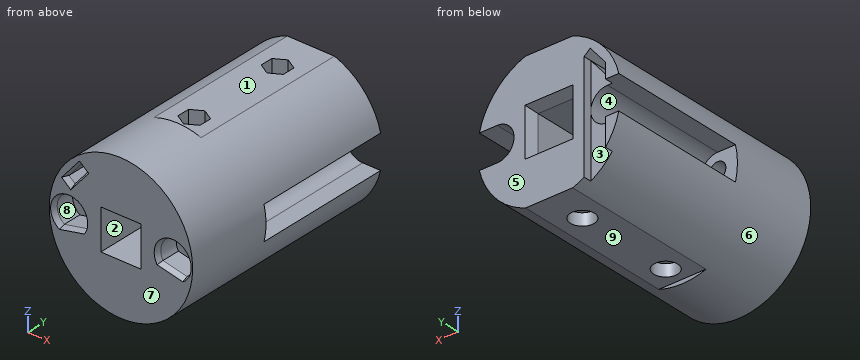
```python
from build123d import *

# Parameters (mm, degrees)
SKETCH1_R           = 18
SKETCH1_R_2         = 2.1
SKETCH1_W           = 10.1
SKETCH1_H           = 10.1
BOSS_EXTRUDE1_DEPTH = 57
CUT_EXTRUDE4_DEPTH  = 40
SKETCH6_R           = 1.5
CUT_EXTRUDE5_DEPTH  = 36
SKETCH7_R           = 3
CUT_EXTRUDE6_DEPTH  = 3
CUT_EXTRUDE7_DEPTH  = 4
CHAMFER1_SIZE       = 1
CHAMFER1_SIZE2      = 2.747477419
CUT_EXTRUDE9_DEPTH  = 6
CHAMFER2_SIZE       = 0.5
CHAMFER2_SIZE2      = 1.37373871
CUT_EXTRUDE10_DEPTH = 35
CUT_EXTRUDE11_DEPTH = 58
CHAMFER3_SIZE       = 0.5
CHAMFER3_SIZE2      = 1.37373871
CUT_EXTRUDE13_DEPTH = 2


with BuildPart() as part:
    # Sketch1 → Boss-Extrude1 (new body)
    with BuildSketch(Plane(origin=(0, 0, 0), x_dir=(1, 0, 0), z_dir=(0, 1, 0))):
        Circle(SKETCH1_R)
        with Locations((13, 0)):
            Circle(SKETCH1_R_2, mode=Mode.SUBTRACT)
        with Locations((-13, 0)):
            Circle(SKETCH1_R_2, mode=Mode.SUBTRACT)
        Rectangle(SKETCH1_W, SKETCH1_H, mode=Mode.SUBTRACT)
    extrude(amount=BOSS_EXTRUDE1_DEPTH)

    # Sketch5 → Cut-Extrude4 (cut)
    with BuildSketch(Plane(origin=(0, 57, 0), x_dir=(1, 0, 0), z_dir=(0, 1, 0))):
        with BuildLine():
            Line((5.916079783, 17), (-5.916079783, 17))
            ThreePointArc((-5.916079783, 17), (0, 18), (5.916079783, 17))
        make_face()
        with BuildLine():
            Line((5.916079783, -17), (-5.916079783, -17))
            ThreePointArc((-5.916079783, -17), (0, -18), (5.916079783, -17))
        make_face()
    extrude(amount=-CUT_EXTRUDE4_DEPTH, mode=Mode.SUBTRACT)

    # Sketch6 → Cut-Extrude5 (cut, through all)
    with BuildSketch(Plane(origin=(0, 0, -17), x_dir=(-1, 0, 0), z_dir=(0, 0, -1))):
        with Locations((0, 47)):
            Circle(SKETCH6_R)
        with Locations((0, 22)):
            Circle(SKETCH6_R)
    extrude(amount=-CUT_EXTRUDE5_DEPTH, mode=Mode.SUBTRACT)

    # Sketch7 → Cut-Extrude6 (cut)
    with BuildSketch(Plane(origin=(0, 0, -17), x_dir=(-1, 0, 0), z_dir=(0, 0, -1))):
        with Locations((0, 47)):
            Circle(SKETCH7_R)
        with Locations((0, 22)):
            Circle(SKETCH7_R)
    extrude(amount=-CUT_EXTRUDE6_DEPTH, mode=Mode.SUBTRACT)

    # Sketch8 → Cut-Extrude7 (cut)
    with BuildSketch(Plane.XY.offset(17)):
        Polygon((0, 43.8), (2.771281292, 45.4), (2.771281292, 48.6), (0, 50.2), (-2.771281292, 48.6), (-2.771281292, 45.4), align=None)
        Polygon((0, 18.8), (2.771281292, 20.4), (2.771281292, 23.6), (0, 25.2), (-2.771281292, 23.6), (-2.771281292, 20.4), align=None)
    extrude(amount=-CUT_EXTRUDE7_DEPTH, mode=Mode.SUBTRACT)

    # Chamfer1
    chamfer1_edges = [part.edges().sort_by_distance(p)[0] for p in [
        (0, 57, -5.05),
        (-5.05, 57, 0),
        (0, 57, 5.05),
        (5.05, 57, 0),
    ]]
    chamfer1_side = [part.faces().sort_by_distance(p)[0] for p in [
        (14.267618119, 57, 10.141691708),
    ]]
    chamfer(chamfer1_edges, length=CHAMFER1_SIZE, length2=CHAMFER1_SIZE2, reference=chamfer1_side[0])

    # Sketch9 → Cut-Extrude9 (cut)
    with BuildSketch(Plane.XZ):
        with BuildLine():
            Line((15.438263477, -3.358179747), (9.406640719, -2.076118753))
            ThreePointArc((9.406640719, -2.076118753), (13.862833517, 4.059312543), (15.438263477, -3.358179747))
        make_face()
        with BuildLine():
            Line((-9.458796565, -2.163880365), (-15.354920877, -3.417140276))
            ThreePointArc((-15.354920877, -3.417140276), (-13.862833517, 4.059312543), (-9.458796565, -2.163880365))
        make_face()
    extrude(amount=-CUT_EXTRUDE9_DEPTH, mode=Mode.SUBTRACT)

    # Chamfer2
    chamfer2_edges = [part.edges().sort_by_distance(p)[0] for p in [
        (13.862833517, 0, 4.059312543),
        (12.422452098, 0, -2.71714925),
        (-13.862833517, 0, 4.059312543),
        (-12.406858721, 0, -2.79051032),
    ]]
    chamfer2_side = [part.faces().sort_by_distance(p)[0] for p in [
        (-17.490883118, 0, 0),
    ]]
    chamfer(chamfer2_edges, length=CHAMFER2_SIZE, length2=CHAMFER2_SIZE2, reference=chamfer2_side[0])

    # Sketch10 → Cut-Extrude10 (cut)
    with BuildSketch(Plane(origin=(0, 57, 0), x_dir=(1, 0, 0), z_dir=(0, 1, 0))):
        with BuildLine():
            Line((13, 4.2), (21, 4.2))
            Line((21, 4.2), (21, -4.2))
            Line((21, -4.2), (13, -4.2))
            ThreePointArc((13, -4.2), (8.8, 0), (13, 4.2))
        make_face()
        with BuildLine():
            Line((-13, 4.2), (-21, 4.2))
            Line((-21, 4.2), (-21, -4.2))
            Line((-21, -4.2), (-13, -4.2))
            ThreePointArc((-13, -4.2), (-8.8, 0), (-13, 4.2))
        make_face()
    extrude(amount=-CUT_EXTRUDE10_DEPTH, mode=Mode.SUBTRACT)

    # Sketch11 → Cut-Extrude11 (cut, through all)
    with BuildSketch(Plane.XZ):
        Polygon((-14.185073919, 7.986468426), (-10.328348261, 12.582735084), (-8.796259375, 11.297159865), (-12.652985033, 6.700893206), align=None)
    extrude(amount=-CUT_EXTRUDE11_DEPTH, mode=Mode.SUBTRACT)

    # Chamfer3
    chamfer3_edges = [part.edges().sort_by_distance(p)[0] for p in [
        (-13.419029476, 0, 7.343680816),
        (-10.724622204, 0, 8.999026536),
        (-9.562303818, 0, 11.939947475),
        (-12.25671109, 0, 10.284601755),
    ]]
    chamfer3_side = [part.faces().sort_by_distance(p)[0] for p in [
        (-17.949088312, 0, 0),
    ]]
    chamfer(chamfer3_edges, length=CHAMFER3_SIZE, length2=CHAMFER3_SIZE2, reference=chamfer3_side[0])

    # Sketch13 → Cut-Extrude13 (cut)
    with BuildSketch(Plane(origin=(0, 57, 0), x_dir=(1, 0, 0), z_dir=(0, 1, 0))):
        with BuildLine():
            Line((-8.796259375, -11.297159865), (-8.796259375, 15.704324914))
            ThreePointArc((-8.796259375, 15.704324914), (-11.720909208, 13.660903606), (-14.185073919, 11.080779662))
            Line((-14.185073919, 11.080779662), (-14.185073919, -7.986468426))
            Line((-14.185073919, -7.986468426), (-8.796259375, -11.297159865))
        make_face()
    extrude(amount=-CUT_EXTRUDE13_DEPTH, mode=Mode.SUBTRACT)


solid = part.part
```
Input: part model. Units: mm. Frame: model coordinates. Face numbers are marked on the shaded views. A direction names the side the tool comes from. Round coordinates to 2 decimals unless told otherwise and drop trailing zeros. Order: outer loops, then holes, each group sorted by start corner. A loop starts at its lowest first (then second) coordinate and runs counter-clockwise, first axis right, second up. Notation, with made-up numbers: (48.5, 32.5) - (74.5, 32.5) arc R15 cw to (74.5, 58.5) - close; hole circle Ø3 at (52, -38.5). An arc over 180 degrees is marked (long way). Answer in a Markdown table with one row per item.
Item 1: Section query B-B (z = 0). Give the number of separate pieces and of enclosed holes in the cut face, then the cut area to 3 significant figures.
Model answer:
| item | result |
|---|---|
| separate pieces | 4 |
| enclosed holes | 0 |
| area | 594 mm² |
Item 2: Mould query, pull axis Z, two halves, no side actions, for the marked faces 6, 7, 8 and 9. Classes: released by +Z, released by -Z, zero draft, split by the parting line, or undercut.
Model answer:
| item | result |
|---|---|
| face 6 | split by the parting line |
| face 7 | zero draft |
| face 8 | undercut |
| face 9 | released by -Z |
Item 3: Pin query (flat end, axial travel): pin 1 (3.5 mm diameter, centred on x = -15.5, y = 47, fed in from -Z); pin 2 (6.5 mm diameter, centred on x = -0.5, y = 47, fed in from -Z); pin 3 (1 mm diameter, centred on y = 56, z = -8, fed in from +X); pin 4 (2.5 mm diameter, centred on x = 0, y = 47, fed in from -Z). Return the tip coordinate at first contact, or that it passes through.
Model answer:
| item | result |
|---|---|
| pin 1 | stops at z = -11.62 |
| pin 2 | stops at z = -17 |
| pin 3 | stops at x = 16.36 |
| pin 4 | passes through |
Item 4: Section query D-D (z = 16). Return the cut outline in (x, y).
Model answer:
| item | result |
|---|---|
| outline | (-8.25, 0) - (8.25, 0) - (8.25, 57) - (-8.25, 57) - close; hole (-2.77, 20.4) - (0, 18.8) - (2.77, 20.4) - (2.77, 23.6) - (0, 25.2) - (-2.77, 23.6) - close; hole (-2.77, 45.4) - (0, 43.8) - (2.77, 45.4) - (2.77, 48.6) - (0, 50.2) - (-2.77, 48.6) - close |
Item 5: Section query A-A (y = 43). Return the cut outline in (x, z).
Model answer:
| item | result |
|---|---|
| outline | (-17.5, -4.2) arc R18 ccw to (-5.92, -17) - (5.92, -17) arc R18 ccw to (17.5, -4.2) - (13, -4.2) arc R4.2 cw to (13, 4.2) - (17.5, 4.2) arc R18 ccw to (5.92, 17) - (-5.92, 17) arc R18 ccw to (-17.5, 4.2) - (-13, 4.2) arc R4.2 cw to (-13, -4.2) - close; hole (-14.19, 7.99) - (-12.65, 6.7) - (-8.8, 11.3) - (-10.33, 12.58) - close; hole (-5.05, -5.05) - (5.05, -5.05) - (5.05, 5.05) - (-5.05, 5.05) - close |
Item 6: Line query: line 1 (Y direction, x = 0, z = -12); line 2 (Z direction, x = 4, y = 53.5); line 3 (Z direction, x = 1, y = 20). Output: solid intervals per line, ascending.
Model answer:
| item | result |
|---|---|
| line 1 | y = 0 to 20.5, 23.5 to 45.5, 48.5 to 57 |
| line 2 | z = -17 to -5.05, 5.05 to 17 |
| line 3 | z = -14 to -5.05, 5.05 to 13 |
Item 7: Reachability of the marked faces 1, 2, 3, 4 and 5 from +Z, -Z, +X, -X, +Y, -Y: full face, straight path, thin tool, end or side. Return the list, or none.
Model answer:
| item | result |
|---|---|
| face 1 | +Z, +X, -X, +Y |
| face 2 | +Y, -Y |
| face 3 | -Z, +Y |
| face 4 | -X, +Y |
| face 5 | +Z, -Z, +X, -X, +Y |
Item 8: Section query C-C (y = 10). Return the cut outline in (x, z), then the cut area to 3 significant figures.
Model answer:
| item | result |
|---|---|
| outline | circle Ø36 at (0, 0); hole circle Ø4.2 at (-13, 0); hole (-14.19, 7.99) - (-12.65, 6.7) - (-8.8, 11.3) - (-10.33, 12.58) - close; hole (-5.05, -5.05) - (5.05, -5.05) - (5.05, 5.05) - (-5.05, 5.05) - close; hole circle Ø4.2 at (13, 0) |
| area | 876 mm² |
